from build123d import *

# Parameters (mm, degrees)
CROQUIS1_R              = 32
CROQUIS1_R_2            = 26
SALIENTE_EXTRUIR1_DEPTH = 27
REDONDEO1_R             = 0.762
CROQUIS2_W              = 0.762
CROQUIS2_H              = 0.762
CROQUIS2_H_2            = 1.27
CROQUIS2_W_2            = 0.381
CROQUIS2_H_3            = 0.508
FILLET1_R               = 1


with BuildPart() as part:
    # Croquis1 → Saliente-Extruir1 (new body)
    with BuildSketch(Plane.XY):
        Circle(CROQUIS1_R)
        Circle(CROQUIS1_R_2, mode=Mode.SUBTRACT)
    extrude(amount=-SALIENTE_EXTRUIR1_DEPTH)

    # Redondeo1
    redondeo1_edges = [part.edges().sort_by_distance(p)[0] for p in [
        (-32, 0, 0),
        (-32, 0, -27),
    ]]
    fillet(redondeo1_edges, radius=REDONDEO1_R)

    # Croquis2 → Cortar-Revolución1 (revolve, cut)
    with BuildSketch(Plane(origin=(0, 0, 0), x_dir=(1, 0, 0), z_dir=(0, 1, 0)), mode=Mode.PRIVATE) as cortar_revoluci_n1_sk:
        with Locations((-31.619, 22.987)):
            Rectangle(CROQUIS2_W, CROQUIS2_H)
        with Locations((-31.619, 18.161)):
            Rectangle(CROQUIS2_W, CROQUIS2_H_2)
        with Locations((-31.8095, 24.892)):
            Rectangle(CROQUIS2_W_2, CROQUIS2_H_3)
        with Locations((-31.619, 9.779)):
            Rectangle(CROQUIS2_W, CROQUIS2_H_2)
        with Locations((-31.619, 4.953)):
            Rectangle(CROQUIS2_W, CROQUIS2_H)
        with Locations((-31.8095, 3.048)):
            Rectangle(CROQUIS2_W_2, CROQUIS2_H_3)
    revolve(cortar_revoluci_n1_sk.sketch.rotate(Axis((0, 0, 0), (0, 0, -1)), 180), axis=Axis((0, 0, 0), (0, 0, -1)), mode=Mode.SUBTRACT)

    # Fillet1
    fillet1_edges = [part.edges().sort_by_distance(p)[0] for p in [
        (-26, 0, 0),
    ]]
    fillet(fillet1_edges, radius=FILLET1_R)


solid = part.part
Model file for the job. Use its own axes, mm. A direction names the side the tool comes from. Give positions to 0.01 mm unless a question says otherwise; leave off trailing zeros. Order: outer loops, then holes, each group sorted by start corner. A loop starts at its lowest first (then second) coordinate and runs counter-clockwise, first axis right, second up. Notation, with made-up numbers: M 42,50.5 L 70,50.5 A20 ccw 70,78.5 Z; hole C -27,36 d1. An arc over 180 degrees is marked long. Put each result on its own line as item: value. Start each with the question number.
(1) Pull direction X, two halves, no side cores. Call faces 1 (the face through (-6.94, -31.24, -3.93)), 2 (the face through (-20.633, -15.821, -13.818)), 3 (the face through (7, 31, -22.606)): released by +X, released by -X, zero draft, split by the parting line, or undercut.
(2) Band-saw the part on A-A on z = -13.5. Give the cut face in (x, y).
(3) Pin check, flat tips, straight feed: pin 1 Ø3 at (y, z) = (23, -18) entering from -X; pin 2 Ø12 at (y, z) = (-22, -18) entering from +X; pin 3 Ø1 at (y, z) = (-19.5, -10) entering from -X; pin 4 Ø19 at (x, y) = (-5.5, -14.5) entering from +Z. Stop position of each tip, or through.
(4) Drill centre lines: L1, parallel to Y at x = 0, z = -13.25; L2, parallel to Y at x = 0, z = -9.75; L3, parallel to X at y = 1.5, z = -8. Where is each one in solid material? Low to high. Write a range as [from, to].
(5) Tool access for faces 4 (the face through (14.414, 27.713, -18.17)), 5 (the face through (-7, 26, -27)): list every direction of +Z, -Z, +X, -X, +Y, -Y with a clear straight run to the whole face (end or side of a thin tool).
Results below:
1. face 1: split by the parting line
1. face 2: undercut
1. face 3: zero draft
2. outline: C 0,0 d64; hole C 0,0 d52
3. pin 1: stops at x = -23.63
3. pin 2: stops at x = 27.7
3. pin 3: stops at x = -25.59
3. pin 4: passes through
4. L1: y = [-32, -26], [26, 32]
4. L2: y = [-31.24, -26], [26, 31.24]
4. L3: x = [-31.96, -25.96], [25.96, 31.96]
5. face 4: none
5. face 5: -Z, +X, -X, +Y, -Y
